Verification items for the finished model (mm, model axes). Round coordinates to 2 decimals unless told otherwise and drop trailing zeros. Loops run counter-clockwise (first coordinate to the right, second up) from the corner with the lowest first, then second, coordinate; pieces in that order, holes last. Notation, with made-up numbers: (-16, 88.5) - (-8, 88.5) arc R20 cw to (-8, 109.5) - close; hole circle Ø6 at (26.25, 54.5). An arc over 180 degrees is marked (long way). Use a Markdown table: item, result. Add a question column.
```python
from build123d import *

# Parameters (mm, degrees)
F0_W     = 47.759749
F0_H     = 32.863535
F1_DEPTH = 25.4
F3_D     = 6.35


with BuildPart() as f1:
    # F0 (on Right) → F1 (new body)
    with BuildSketch(Plane.YZ):
        with Locations((23.879874, 16.431767)):
            Rectangle(F0_W, F0_H)
    extrude(amount=F1_DEPTH)

    # F3 (through all)
    with Locations(Plane.YZ.offset(25.4)):
        with Locations((24.755191, 18.47573)):
            Hole(F3_D / 2)


solid = f1.part
```
Q1. Thickness scan on line 1 along Z through (x, y) = (15, 24.5); line 2 along Z through (x, y) = (13.5, 23). Record the ranges inside material, lowest first.
Q2. Section check B-B on x = 16.5. Record the cut outline in (y, z) (3 decimals), plus the area to 3 significant figures.
Q3. Release check for a two-part mould opening along Y. For faces 1 (the face through (13, 47.76, 16)), 2 (the face through (13, 24, 0)), 3 (the face through (12.522, 25.169, 21.624)) record: +Y half, -Y half, draft (parallel to the pull), parting line (faces both ways), or undercut.
Q4. Section check A-A on y = 24. Record the cut outline in (x, z).
Determined:
| question | item | result |
|---|---|---|
| 1 | line 1 | z = 0 to 15.31, 21.64 to 32.86 |
| 1 | line 2 | z = 0 to 15.83, 21.12 to 32.86 |
| 2 | outline | (0, 0) - (47.76, 0) - (47.76, 32.864) - (0, 32.864) - close; hole circle Ø6.35 at (24.755, 18.476) |
| 2 | area | 1,540 mm² |
| 3 | face 1 | +Y half |
| 3 | face 2 | draft |
| 3 | face 3 | undercut |
| 4 | outline | (0, 0) - (25.4, 0) - (25.4, 15.39) - (0, 15.39) - close; (0, 21.56) - (25.4, 21.56) - (25.4, 32.86) - (0, 32.86) - close |
